Source: CAD feature listing. Evaluate the final solid. Frame: model axes, mm. Give positions to 0.01 mm unless a question says otherwise; leave off trailing zeros. Order: outer loops, then holes, each group sorted by start corner. A loop starts at its lowest first (then second) coordinate and runs counter-clockwise, first axis right, second up. Notation, with made-up numbers: M 16,26.25 L 74,26.25 A11 cw 74,37.25 Z; hole C -34.5,63.25 d1. An arc over 180 degrees is marked long. Return JSON: item names as keys, results as strings.
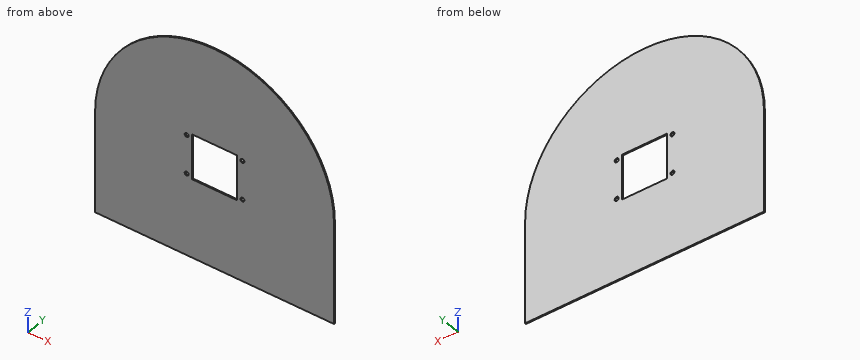
from build123d import *

# Parameters (mm, degrees)
F0_R     = 5
F1_DEPTH = 3


with BuildPart() as f1:
    # F0 (on Front) → F1 (new body)
    with BuildSketch(Plane.XZ):
        with BuildLine():
            ThreePointArc((75, 79), (70, 84), (65, 79))
            ThreePointArc((65, 79), (70, 74), (75, 79))
        make_face()
        with Locations((-70, 79)):
            Circle(F0_R)
        Polygon((-300, 128), (-300, -128), (300, -128), (300, 128), (57, 128), (57, 79), (57, 71), (-57, 71), (-57, 79), (-57, 128), align=None)
        with Locations((-70, 79)):
            Circle(F0_R, mode=Mode.SUBTRACT)
        with BuildLine():
            ThreePointArc((75, 79), (70, 74), (65, 79))
            ThreePointArc((65, 79), (70, 84), (75, 79))
        make_face(mode=Mode.SUBTRACT)
        with Locations((-70, 177)):
            Circle(F0_R)
        with BuildLine():
            ThreePointArc((75, 177), (70, 182), (65, 177))
            ThreePointArc((65, 177), (70, 172), (75, 177))
        make_face()
        with BuildLine():
            ThreePointArc((300, 128), (0, 428), (-300, 128))
            Line((-300, 128), (-57, 128))
            Line((-57, 128), (-57, 177))
            Line((-57, 177), (-57, 185))
            Line((-57, 185), (57, 185))
            Line((57, 185), (57, 177))
            Line((57, 177), (57, 128))
            Line((57, 128), (300, 128))
        make_face()
        with Locations((-70, 177)):
            Circle(F0_R, mode=Mode.SUBTRACT)
        with BuildLine():
            ThreePointArc((75, 177), (70, 172), (65, 177))
            ThreePointArc((65, 177), (70, 182), (75, 177))
        make_face(mode=Mode.SUBTRACT)
    extrude(amount=F1_DEPTH)


solid = f1.part
1. Section query C-C (y = -0.85). Return loops of the section in (x, z), then the cut area to 3 significant figures.
Evaluation:
{"outline": "M -300,-128 L 300,-128 L 300,128 A300 ccw -300,128 Z; hole C -70,79 d10; hole C -70,177 d10; hole M -57,71 L 57,71 L 57,185 L -57,185 Z; hole C 70,79 d10; hole C 70,177 d10", "area": "282,000 mm^2"}
2. Section query B-B (z = 97). Return loops of the section in (x, y), then the cut area to 3 significant figures.
Evaluation:
{"outline": "M -300,-3 L -57,-3 L -57,0 L -300,0 Z; M 57,-3 L 300,-3 L 300,0 L 57,0 Z", "area": "1,460 mm^2"}
3. Section query A-A (x = 0). Return loops of the section in (y, z), then the cut area to 3 significant figures.
Evaluation:
{"outline": "M -3,-128 L 0,-128 L 0,71 L -3,71 Z; M -3,185 L 0,185 L 0,428 L -3,428 Z", "area": "1,330 mm^2"}
4. Ray query, probe 1 along Z at (x, y) = (-70, -1.8); probe 2 along Z at (x, y) = (-18.5, -0.2); probe 3 along Z at (x, y) = (-26, -0.8). Return the intervals inside material, ascending.
Evaluation:
{"probe 1": "z = -128 to 74, 84 to 172, 182 to 419.72", "probe 2": "z = -128 to 71, 185 to 427.43", "probe 3": "z = -128 to 71, 185 to 426.87"}
5. Section query D-D (x = -165). Return loops of the section in (y, z).
Evaluation:
{"outline": "M -3,-128 L 0,-128 L 0,378.55 L -3,378.55 Z"}
6. First-contact query: pin 1 (1.5 mm diameter, centred on y = -1, z = 354.5, fed in from -X); pin 2 (12 mm diameter, centred on x = 61, z = 114.5, fed in from +Y); pin 3 (6 mm diameter, centred on x = -70, z = 177, fed in from +Y). Flat tips, straight axial feed; report the tip coordinate or a pass-through.
Evaluation:
{"pin 1": "stops at x = -197.58", "pin 2": "stops at y = 0", "pin 3": "passes through"}
